```python
from build123d import *

# Parameters (mm, degrees)
BOSS_EXTRUDE1_DEPTH                             = 8.5
SKETCH5_W                                       = 36
SKETCH5_H                                       = 8.5
BOSS_EXTRUDE2_DEPTH                             = 100
CSK_FOR_M3_FLAT_HEAD_MACHINE_SCREW2_D           = 3.4
CSK_FOR_M3_FLAT_HEAD_MACHINE_SCREW2_DEPTH       = 10
CSK_FOR_M3_FLAT_HEAD_MACHINE_SCREW2_CSINK_D     = 6.3
CSK_FOR_M3_FLAT_HEAD_MACHINE_SCREW2_CSINK_ANGLE = 90
CSK_FOR_M3_FLAT_HEAD_MACHINE_SCREW2_TIP         = 1.021463052
LPATTERN1_COUNT                                 = 12
LPATTERN1_PITCH                                 = 8


with BuildPart() as part:
    # Sketch1 → Boss-Extrude1 (new body)
    with BuildSketch(Plane.XY):
        with BuildLine():
            Line((0, 0), (48, 0))
            ThreePointArc((48, 0), (46.242640687, 4.242640687), (42, 6))
            Line((42, 6), (6, 6))
            ThreePointArc((6, 6), (1.757359313, 4.242640687), (0, 0))
        make_face()
    extrude(amount=BOSS_EXTRUDE1_DEPTH)

    # Sketch5 → Boss-Extrude2 (add)
    with BuildSketch(Plane(origin=(0, 6, 0), x_dir=(1, 0, 0), z_dir=(0, 1, 0))):
        with Locations((24, -4.25)):
            Rectangle(SKETCH5_W, SKETCH5_H)
    extrude(amount=BOSS_EXTRUDE2_DEPTH)

    # Sketch14 → Ø3.0mm Dowel Hole3 (revolve, cut)
    with BuildSketch(Plane(origin=(37, 101, 0), x_dir=(0, 1, 0), z_dir=(1, 0, 0))):
        Polygon((0, 0), (0, 5.901290929), (1.5, 5), (1.5, 0), align=None)
    f_3_0mm_dowel_hole3 = revolve(axis=Axis((37, 101, -6.35), (0, 0, 1)), mode=Mode.SUBTRACT)

    # CSK for M3 Flat Head Machine Screw2
    with Locations(Plane(origin=(0, 0, 0), x_dir=(-1, 0, 0), z_dir=(0, -1, 0))):
        with Locations((-39, -4.25), (-9, -4.25)):
            CounterSinkHole(CSK_FOR_M3_FLAT_HEAD_MACHINE_SCREW2_D / 2, CSK_FOR_M3_FLAT_HEAD_MACHINE_SCREW2_CSINK_D / 2, depth=CSK_FOR_M3_FLAT_HEAD_MACHINE_SCREW2_DEPTH, counter_sink_angle=CSK_FOR_M3_FLAT_HEAD_MACHINE_SCREW2_CSINK_ANGLE)
            with Locations((0, 0, -(CSK_FOR_M3_FLAT_HEAD_MACHINE_SCREW2_DEPTH + CSK_FOR_M3_FLAT_HEAD_MACHINE_SCREW2_TIP / 2))):  # 118° drill point
                Cone(0, CSK_FOR_M3_FLAT_HEAD_MACHINE_SCREW2_D / 2, CSK_FOR_M3_FLAT_HEAD_MACHINE_SCREW2_TIP, mode=Mode.SUBTRACT)

    # Mirror1: Ø3.0mm Dowel Hole3 across plane
    add(f_3_0mm_dowel_hole3.mirror(Plane(origin=(24, 0, 0), x_dir=(0, 0, 1), z_dir=(1, 0, 0))), mode=Mode.SUBTRACT)

    # LPattern1: Ø3.0mm Dowel Hole3 ×12
    with Locations(*[(0, -i * LPATTERN1_PITCH, 0) for i in range(1, LPATTERN1_COUNT)]):
        add(f_3_0mm_dowel_hole3, mode=Mode.SUBTRACT)

    # LPattern1 copy 1 sketch → LPattern1 copy 1 (revolve, cut)
    with BuildSketch(Plane(origin=(11, 93, 0), x_dir=(0, 1, 0), z_dir=(-1, 0, 0))):
        Polygon((0, 0), (0, -5.901290929), (1.5, -5), (1.5, 0), align=None)
    revolve(axis=Axis((11, 93, -6.35), (0, 0, -1)), mode=Mode.SUBTRACT)

    # LPattern1 copy 2 sketch → LPattern1 copy 2 (revolve, cut)
    with BuildSketch(Plane(origin=(11, 85, 0), x_dir=(0, 1, 0), z_dir=(-1, 0, 0))):
        Polygon((0, 0), (0, -5.901290929), (1.5, -5), (1.5, 0), align=None)
    revolve(axis=Axis((11, 85, -6.35), (0, 0, -1)), mode=Mode.SUBTRACT)

    # LPattern1 copy 3 sketch → LPattern1 copy 3 (revolve, cut)
    with BuildSketch(Plane(origin=(11, 77, 0), x_dir=(0, 1, 0), z_dir=(-1, 0, 0))):
        Polygon((0, 0), (0, -5.901290929), (1.5, -5), (1.5, 0), align=None)
    revolve(axis=Axis((11, 77, -6.35), (0, 0, -1)), mode=Mode.SUBTRACT)

    # LPattern1 copy 4 sketch → LPattern1 copy 4 (revolve, cut)
    with BuildSketch(Plane(origin=(11, 69, 0), x_dir=(0, 1, 0), z_dir=(-1, 0, 0))):
        Polygon((0, 0), (0, -5.901290929), (1.5, -5), (1.5, 0), align=None)
    revolve(axis=Axis((11, 69, -6.35), (0, 0, -1)), mode=Mode.SUBTRACT)

    # LPattern1 copy 5 sketch → LPattern1 copy 5 (revolve, cut)
    with BuildSketch(Plane(origin=(11, 61, 0), x_dir=(0, 1, 0), z_dir=(-1, 0, 0))):
        Polygon((0, 0), (0, -5.901290929), (1.5, -5), (1.5, 0), align=None)
    revolve(axis=Axis((11, 61, -6.35), (0, 0, -1)), mode=Mode.SUBTRACT)

    # LPattern1 copy 6 sketch → LPattern1 copy 6 (revolve, cut)
    with BuildSketch(Plane(origin=(11, 53, 0), x_dir=(0, 1, 0), z_dir=(-1, 0, 0))):
        Polygon((0, 0), (0, -5.901290929), (1.5, -5), (1.5, 0), align=None)
    revolve(axis=Axis((11, 53, -6.35), (0, 0, -1)), mode=Mode.SUBTRACT)

    # LPattern1 copy 7 sketch → LPattern1 copy 7 (revolve, cut)
    with BuildSketch(Plane(origin=(11, 45, 0), x_dir=(0, 1, 0), z_dir=(-1, 0, 0))):
        Polygon((0, 0), (0, -5.901290929), (1.5, -5), (1.5, 0), align=None)
    revolve(axis=Axis((11, 45, -6.35), (0, 0, -1)), mode=Mode.SUBTRACT)

    # LPattern1 copy 8 sketch → LPattern1 copy 8 (revolve, cut)
    with BuildSketch(Plane(origin=(11, 37, 0), x_dir=(0, 1, 0), z_dir=(-1, 0, 0))):
        Polygon((0, 0), (0, -5.901290929), (1.5, -5), (1.5, 0), align=None)
    revolve(axis=Axis((11, 37, -6.35), (0, 0, -1)), mode=Mode.SUBTRACT)

    # LPattern1 copy 9 sketch → LPattern1 copy 9 (revolve, cut)
    with BuildSketch(Plane(origin=(11, 29, 0), x_dir=(0, 1, 0), z_dir=(-1, 0, 0))):
        Polygon((0, 0), (0, -5.901290929), (1.5, -5), (1.5, 0), align=None)
    revolve(axis=Axis((11, 29, -6.35), (0, 0, -1)), mode=Mode.SUBTRACT)

    # LPattern1 copy 10 sketch → LPattern1 copy 10 (revolve, cut)
    with BuildSketch(Plane(origin=(11, 21, 0), x_dir=(0, 1, 0), z_dir=(-1, 0, 0))):
        Polygon((0, 0), (0, -5.901290929), (1.5, -5), (1.5, 0), align=None)
    revolve(axis=Axis((11, 21, -6.35), (0, 0, -1)), mode=Mode.SUBTRACT)

    # LPattern1 copy 11 sketch → LPattern1 copy 11 (revolve, cut)
    with BuildSketch(Plane(origin=(11, 13, 0), x_dir=(0, 1, 0), z_dir=(-1, 0, 0))):
        Polygon((0, 0), (0, -5.901290929), (1.5, -5), (1.5, 0), align=None)
    revolve(axis=Axis((11, 13, -6.35), (0, 0, -1)), mode=Mode.SUBTRACT)


solid = part.part
```
For this review, take the finished solid that the model builds, in its own axes (mm). A direction names the side the tool comes from. Coordinates: 2 decimals unless noted, no trailing zeros. Order: outer loops, then holes, each group sorted by start corner. A loop starts at its lowest first (then second) coordinate and runs counter-clockwise, first axis right, second up. Notation, with made-up numbers: (-24, -15) - (-11, -15) arc R31 cw to (-11, 11) - close; hole circle Ø4 at (-28, -7). An arc over 180 degrees is marked (long way). Answer as a JSON object with one key per item and string values. Group by question number.
1. The part is to be moulded in two halves that separate along Y. For faces 1 (the cylindrical face through (12.265, 101.806, 2.465)), 2 (the flat face through (6, 55, 4)), 3 (the conical face through (8.718, 10.844, 4.161)), 4 (the cylindrical face through (1.804, 4.289, 4.19)), say which applies: pulls with the +Y half, pulls with the -Y half, needs draft (parallel to the pull), parting line crosses it, or undercut.
2. For faces 5 (the flat face through (42, 55, 4)), 6 (the flat face through (24, 106, 4)), 7 (the cylindrical face through (37.9, 43.8, 2.5)), list the 3-axis set-ups (+Z, -Z, +X, -X, +Y, -Y) from which the entire face can be reached by the end or side of a thin tool; tool diameter is ignored.
3. We need section B-B on x = 45. State the section outline as (y, z) points, then the cut area to 3 significant figures.
4. We need section A-A on y = 32. State the section outline as (x, z) points, then the cut area to 3 significant figures.
5. Clearance check with flat-ended pins moving along their axes: P1, Ø2.5, axis at y = 40.5, z = 4, coming from the -X side; P2, Ø2.5, axis at x = 9, z = 4.25, coming from the -Y side; P3, Ø1.8, axis at x = 37, y = 29, coming from the -Z side. State where each tip first meets the part, or that it passes through.
6. For probe 1 along X at (y, z) = (61, 2.5); probe 2 along Z at (x, y) = (9, 5); probe 3 along X at (y, z) = (8.5, 5.5), list the stretches that pass through material, from the lowest coordinate up.
Final values:
{
 "1": {"face 1": "undercut", "face 2": "needs draft", "face 3": "pulls with the -Y half", "face 4": "pulls with the +Y half"},
 "2": {"face 5": "+Z, -Z, +X, +Y", "face 6": "+Z, -Z, +X, -X, +Y", "face 7": "-Z"},
 "3": {"outline": "(0, 0) - (5.2, 0) - (5.2, 8.5) - (0, 8.5) - close", "area": "44.2 mm²"},
 "4": {"outline": "(6, 0) - (42, 0) - (42, 8.5) - (6, 8.5) - close", "area": "306 mm²"},
 "5": {"P1": "x = 6", "P2": "y = 10.27", "P3": "z = 5.36"},
 "6": {"probe 1": "6 to 9.5, 12.5 to 35.5, 38.5 to 42", "probe 2": "0 to 2.55, 5.95 to 8.5", "probe 3": "6 to 7.85, 10.15 to 37.85, 40.15 to 42"}
}
